from build123d import *

# Parameters (mm, degrees)
ESQUISSE1_W        = 160
ESQUISSE1_H        = 60
BOSS_EXTRU_1_DEPTH = 30
ESQUISSE2_W        = 4
ESQUISSE2_H        = 4
BOSS_EXTRU_2_DEPTH = 5
CONG_1_R           = 10


with BuildPart() as part:
    # Esquisse1 → Boss.-Extru.1 (new body)
    with BuildSketch(Plane(origin=(0, 0, 0), x_dir=(1, 0, 0), z_dir=(0, 1, 0))):
        Rectangle(ESQUISSE1_W, ESQUISSE1_H)
    extrude(amount=BOSS_EXTRU_1_DEPTH)

    # Esquisse2 → Boss.-Extru.2 (add)
    with BuildSketch(Plane(origin=(80, 0, 0), x_dir=(0, 0, -1), z_dir=(1, 0, 0))):
        with Locations((25.192260315, 18)):
            Rectangle(ESQUISSE2_W, ESQUISSE2_H)
        with Locations((25.192260315, 12)):
            Rectangle(ESQUISSE2_W, ESQUISSE2_H)
    extrude(amount=BOSS_EXTRU_2_DEPTH)

    # Congé1
    # the kernel refuses this fillet: 10 mm, written as the material it takes off along each edge
    with BuildSketch(Plane(origin=(-70, 20, 20), x_dir=(-1, 0, 0), z_dir=(0, 0, 1))) as cong_1_piece_1_section:
        Polygon((0, 0), (CONG_1_R * 1.02, 0), (CONG_1_R * 1.02, -CONG_1_R * 1.02), (0, -CONG_1_R * 1.02), align=None)
    cong_1_piece_1 = extrude(amount=CONG_1_R * 1.02, mode=Mode.PRIVATE)
    cong_1_piece_1 = cong_1_piece_1 - Plane(origin=(-70, 20, 20), x_dir=(0.7071067811865475, -0.7071067811865475, 0), z_dir=(0, 0, 1)) * Sphere(CONG_1_R, mode=Mode.PRIVATE)
    add(cong_1_piece_1, mode=Mode.SUBTRACT)
    with BuildSketch(Plane(origin=(-70, 20, -20), x_dir=(0, 1, 0), z_dir=(-1, 0, 0))) as cong_1_piece_2_section:
        Polygon((0, 0), (CONG_1_R * 1.02, 0), (CONG_1_R * 1.02, CONG_1_R * 1.02), (0, CONG_1_R * 1.02), align=None)
    cong_1_piece_2 = extrude(amount=CONG_1_R * 1.02, mode=Mode.PRIVATE)
    cong_1_piece_2 = cong_1_piece_2 - Plane(origin=(-70, 20, -20), x_dir=(0, -0.7071067811865475, 0.7071067811865475), z_dir=(-1, 0, 0)) * Sphere(CONG_1_R, mode=Mode.PRIVATE)
    add(cong_1_piece_2, mode=Mode.SUBTRACT)
    with BuildSketch(Plane(origin=(70, 10, -20), x_dir=(0, -1, 0), z_dir=(1, 0, 0))) as cong_1_piece_3_section:
        Polygon((0, 0), (CONG_1_R * 1.02, 0), (CONG_1_R * 1.02, CONG_1_R * 1.02), (0, CONG_1_R * 1.02), align=None)
    cong_1_piece_3 = extrude(amount=CONG_1_R * 1.02, mode=Mode.PRIVATE)
    cong_1_piece_3 = cong_1_piece_3 - Plane(origin=(70, 10, -20), x_dir=(0, 0.7071067811865475, 0.7071067811865475), z_dir=(1, 0, 0)) * Sphere(CONG_1_R, mode=Mode.PRIVATE)
    add(cong_1_piece_3, mode=Mode.SUBTRACT)
    with BuildSketch(Plane(origin=(70, 20, -20), x_dir=(0, 1, 0), z_dir=(1, 0, 0))) as cong_1_piece_4_section:
        Polygon((0, 0), (CONG_1_R * 1.02, 0), (CONG_1_R * 1.02, -CONG_1_R * 1.02), (0, -CONG_1_R * 1.02), align=None)
    cong_1_piece_4 = extrude(amount=CONG_1_R * 1.02, mode=Mode.PRIVATE)
    cong_1_piece_4 = cong_1_piece_4 - Plane(origin=(70, 20, -20), x_dir=(0, -0.7071067811865475, 0.7071067811865475), z_dir=(1, 0, 0)) * Sphere(CONG_1_R, mode=Mode.PRIVATE)
    add(cong_1_piece_4, mode=Mode.SUBTRACT)
    with BuildSketch(Plane(origin=(70, 10, 20), x_dir=(1, 0, 0), z_dir=(0, 0, 1))) as cong_1_piece_5_section:
        Polygon((0, 0), (CONG_1_R * 1.02, 0), (CONG_1_R * 1.02, -CONG_1_R * 1.02), (0, -CONG_1_R * 1.02), align=None)
    cong_1_piece_5 = extrude(amount=CONG_1_R * 1.02, mode=Mode.PRIVATE)
    cong_1_piece_5 = cong_1_piece_5 - Plane(origin=(70, 10, 20), x_dir=(-0.7071067811865475, 0.7071067811865475, 0), z_dir=(0, 0, 1)) * Sphere(CONG_1_R, mode=Mode.PRIVATE)
    add(cong_1_piece_5, mode=Mode.SUBTRACT)
    with BuildSketch(Plane(origin=(70, 20, 20), x_dir=(1, 0, 0), z_dir=(0, 0, 1))) as cong_1_piece_6_section:
        Polygon((0, 0), (CONG_1_R * 1.02, 0), (CONG_1_R * 1.02, CONG_1_R * 1.02), (0, CONG_1_R * 1.02), align=None)
    cong_1_piece_6 = extrude(amount=CONG_1_R * 1.02, mode=Mode.PRIVATE)
    cong_1_piece_6 = cong_1_piece_6 - Plane(origin=(70, 20, 20), x_dir=(-0.7071067811865475, -0.7071067811865475, 0), z_dir=(0, 0, 1)) * Sphere(CONG_1_R, mode=Mode.PRIVATE)
    add(cong_1_piece_6, mode=Mode.SUBTRACT)
    with BuildSketch(Plane(origin=(-80, -25, 30), x_dir=(1, 0, 0), z_dir=(0, 1, 0)), Plane(origin=(-80, -25, -30), x_dir=(0, 0, 1), z_dir=(0, 1, 0))) as cong_1_piece_7:
        with BuildLine():
            CenterArc((CONG_1_R, CONG_1_R), CONG_1_R, 180, 90)
            Line((0, CONG_1_R), (0, 0))
            Line((0, 0), (CONG_1_R, 0))
        make_face()
    extrude(amount=45, mode=Mode.SUBTRACT)
    with BuildSketch(Plane(origin=(70, 0, -30), x_dir=(0, 0, 1), z_dir=(-1, 0, 0))) as cong_1_piece_8:
        with BuildLine():
            CenterArc((CONG_1_R, CONG_1_R), CONG_1_R, 180, 90)
            Line((0, CONG_1_R), (0, 0))
            Line((0, 0), (CONG_1_R, 0))
        make_face()
    extrude(amount=175, mode=Mode.SUBTRACT)
    with BuildSketch(Plane(origin=(80, 10, -30), x_dir=(0, 0, 1), z_dir=(0, 1, 0))) as cong_1_piece_9_section:
        with BuildLine():
            CenterArc((CONG_1_R, -CONG_1_R), CONG_1_R, 90, 90)
            Line((0, -CONG_1_R), (0, 0))
            Line((0, 0), (CONG_1_R, 0))
        make_face()
    cong_1_piece_9 = extrude(amount=10, mode=Mode.PRIVATE)
    cong_1_piece_9 = split(cong_1_piece_9, bisect_by=Plane(origin=(79.843765754, 12, -23.192260315), z_dir=(0, 0, 1)), keep=Keep.TOP, mode=Mode.PRIVATE)
    add(cong_1_piece_9, mode=Mode.SUBTRACT)
    with BuildSketch(Plane(origin=(80, 10, -30), x_dir=(0, 0, 1), z_dir=(0, 1, 0))) as cong_1_piece_10_section:
        with BuildLine():
            CenterArc((CONG_1_R, -CONG_1_R), CONG_1_R, 90, 90)
            Line((0, -CONG_1_R), (0, 0))
            Line((0, 0), (CONG_1_R, 0))
        make_face()
    cong_1_piece_10 = extrude(amount=10, mode=Mode.PRIVATE)
    cong_1_piece_10 = split(cong_1_piece_10, bisect_by=Plane(origin=(77.140541655, 12, -27.192260315), z_dir=(0, 0, -1)), keep=Keep.TOP, mode=Mode.PRIVATE)
    add(cong_1_piece_10, mode=Mode.SUBTRACT)
    with BuildSketch(Plane(origin=(80, 10, -30), x_dir=(0, 0, 1), z_dir=(0, 1, 0))) as cong_1_piece_11_section:
        with BuildLine():
            CenterArc((CONG_1_R, -CONG_1_R), CONG_1_R, 90, 90)
            Line((0, -CONG_1_R), (0, 0))
            Line((0, 0), (CONG_1_R, 0))
        make_face()
    cong_1_piece_11 = extrude(amount=10, mode=Mode.PRIVATE)
    cong_1_piece_11 = split(cong_1_piece_11, bisect_by=Plane(origin=(79.050284637, 16, -25.722845845), z_dir=(0, -1, 0)), keep=Keep.TOP, mode=Mode.PRIVATE)
    cong_1_piece_11 = split(cong_1_piece_11, bisect_by=Plane(origin=(79.050284637, 14, -25.722845845), z_dir=(0, 1, 0)), keep=Keep.TOP, mode=Mode.PRIVATE)
    add(cong_1_piece_11, mode=Mode.SUBTRACT)
    with BuildSketch(Plane(origin=(80, 0, 20), x_dir=(0, 1, 0), z_dir=(0, 0, -1))) as cong_1_piece_12:
        with BuildLine():
            CenterArc((CONG_1_R, -CONG_1_R), CONG_1_R, 90, 90)
            Line((0, -CONG_1_R), (0, 0))
            Line((0, 0), (CONG_1_R, 0))
        make_face()
    extrude(amount=40, mode=Mode.SUBTRACT)
    with BuildSketch(Plane(origin=(80, 30, 20), x_dir=(0, -1, 0), z_dir=(0, 0, -1)), Plane(origin=(-80, 30, -20), x_dir=(0, -1, 0), z_dir=(0, 0, 1))) as cong_1_piece_13:
        with BuildLine():
            CenterArc((CONG_1_R, CONG_1_R), CONG_1_R, 180, 90)
            Line((0, CONG_1_R), (0, 0))
            Line((0, 0), (CONG_1_R, 0))
        make_face()
    extrude(amount=40, mode=Mode.SUBTRACT)
    with BuildSketch(Plane(origin=(70, 30, -30), x_dir=(0, 0, 1), z_dir=(-1, 0, 0))) as cong_1_piece_14:
        with BuildLine():
            CenterArc((CONG_1_R, -CONG_1_R), CONG_1_R, 90, 90)
            Line((0, -CONG_1_R), (0, 0))
            Line((0, 0), (CONG_1_R, 0))
        make_face()
    extrude(amount=140, mode=Mode.SUBTRACT)
    with BuildSketch(Plane(origin=(80, 10, 30), x_dir=(-1, 0, 0), z_dir=(0, 1, 0))) as cong_1_piece_15:
        with BuildLine():
            CenterArc((CONG_1_R, -CONG_1_R), CONG_1_R, 90, 90)
            Line((0, -CONG_1_R), (0, 0))
            Line((0, 0), (CONG_1_R, 0))
        make_face()
    extrude(amount=10, mode=Mode.SUBTRACT)
    with BuildSketch(Plane(origin=(-105, 0, 30), x_dir=(0, 1, 0), z_dir=(1, 0, 0))) as cong_1_piece_16:
        with BuildLine():
            CenterArc((CONG_1_R, -CONG_1_R), CONG_1_R, 90, 90)
            Line((0, -CONG_1_R), (0, 0))
            Line((0, 0), (CONG_1_R, 0))
        make_face()
    extrude(amount=175, mode=Mode.SUBTRACT)
    with BuildSketch(Plane(origin=(-70, 30, 30), x_dir=(0, -1, 0), z_dir=(1, 0, 0))) as cong_1_piece_17:
        with BuildLine():
            CenterArc((CONG_1_R, CONG_1_R), CONG_1_R, 180, 90)
            Line((0, CONG_1_R), (0, 0))
            Line((0, 0), (CONG_1_R, 0))
        make_face()
    extrude(amount=140, mode=Mode.SUBTRACT)


solid = part.part
Read the model definition and answer for the solid it produces. Units are mm, in the model's axes. A direction names the side the tool comes from. Round coordinates to 2 decimals unless told otherwise and drop trailing zeros. Write each loop counter-clockwise with the first axis right and the second up, starting at its lowest first coordinate (ties: lowest second). Pieces come first, ordered by that corner, then holes.
1. The part is cut by section D-D, the plane x = 74.5. Determine the outline of the cut face in (y, z), then the cut area to 3 significant figures.
2. Determine the mould class of faces 6 (the face through (0.98, 27.15, -26.99)), 7 (the face through (-1, 15, -30)), 8 (the face through (82, 14, -25)) for opening direction Y: pulls with the +Y half, pulls with the -Y half, needs draft (parallel to the pull), parting line crosses it, or undercut.
3. Which of the six approach directions +Z, -Z, +X, -X, +Y, -Y give full straight-line access (tool end or side, diameter ignored) to faces 1 (the face through (76.99, 27.15, 0.28)), 2 (the face through (82, 20, -25)), 3 (the face through (-1, 15, 30)), 4 (the face through (80, 15, 0)), 5 (the face through (81, 18, -27.192))?
4. The part is cut by section C-C, the plane z = 17. Determine the outline of the cut face in (x, y).
5. The part is cut by section A-A, the plane y = 18.5. Determine the outline of the cut face in (x, z), then the cut area to 3 significant figures.
6. Given pin 1 Ø10 at (y, z) = (16.5, -7.5) entering from +X; pin 2 Ø4.5 at (x, z) = (80, -25) entering from +Y; pin 3 Ø2 at (x, y) = (82, 12.5) entering from +Z, each flat-ended and moving along its own axis, determine where each tip first touches the part or whether it passes through.
7. Straight lines are drawn through the part: L1, parallel to X at y = 14, z = -6; L2, parallel to Z at x = -62.5, y = 9.5; L3, parallel to X at y = 24.5, z = 7. For each, find the intervals that lie inside material, in ascending order.
8. The part is cut by section B-B, the plane x = -19.5. Determine the outline of the cut face in (y, z), then the cut area to 3 significant figures.
Values:
1. outline: (1.07, -20) arc R8.93 ccw to (10, -28.93) - (20, -28.93) arc R8.93 ccw to (28.93, -20) - (28.93, 20) arc R8.93 ccw to (20, 28.93) - (10, 28.93) arc R8.93 ccw to (1.07, 20) - close
1. area: 1,540 mm2
2. face 6: pulls with the +Y half
2. face 7: needs draft
2. face 8: undercut
3. face 1: +Z, -Z, +X, +Y
3. face 2: -Z, +X, +Y
3. face 3: +Z, +X, -X, +Y, -Y
3. face 4: +Z, +X, +Y, -Y
3. face 5: -Z, +X, +Y, -Y
4. outline: (-80, 0) - (70, 0) arc R10 ccw to (80, 10) - (80, 20) arc R10 ccw to (70, 30) - (-70, 30) arc R10 ccw to (-80, 20) - close
5. outline: (-80, -20) arc R10 ccw to (-70, -30) - (70, -30) arc R10 ccw to (76.95, -27.19) - (85, -27.19) - (85, -23.19) - (79.48, -23.19) arc R10 ccw to (80, -20) - (80, 20) arc R10 ccw to (70, 30) - (-70, 30) arc R10 ccw to (-80, 20) - close
5. area: 9,540 mm2
6. pin 1: stops at x = 80
6. pin 2: stops at y = 24.5
6. pin 3: stops at z = -23.19
7. L1: x = -80 to 80
7. L2: z = -29.99 to 29.99
7. L3: x = -78.93 to 78.93
8. outline: (0, -20) arc R10 ccw to (10, -30) - (20, -30) arc R10 ccw to (30, -20) - (30, 20) arc R10 ccw to (20, 30) - (10, 30) arc R10 ccw to (0, 20) - close
8. area: 1,710 mm2
